```python
from build123d import *

# Parameters (mm, degrees)
REVOLUCI_N1_ANGLE       = 180
CROQUIS2_R              = 19
CORTAR_EXTRUIR1_DEPTH   = 29
SALIENTE_EXTRUIR1_DEPTH = 15
CROQUIS4_W              = 7
CROQUIS4_H              = 28
SALIENTE_EXTRUIR2_DEPTH = 10
CHAFL_N1_SIZE           = 5
REDONDEO1_R             = 10
CORTAR_EXTRUIR2_DEPTH   = 40


with BuildPart() as part:
    # Croquis1 → Revolución1 (revolve)
    with BuildSketch(Plane.XY):
        Polygon((0, 0), (0, 28), (25, 28), (25, 23), (22, 23), (22, 18), (25, 18), (25, 10), (22, 10), (22, 5), (25, 5), (25, 0), align=None)
    revolve(axis=Axis((0, 0, 0), (0, 1, 0)), revolution_arc=REVOLUCI_N1_ANGLE)

    # Croquis2 → Cortar-Extruir1 (cut)
    with BuildSketch(Plane(origin=(0, 28, 0), x_dir=(1, 0, 0), z_dir=(0, 1, 0))):
        Circle(CROQUIS2_R)
    extrude(amount=-CORTAR_EXTRUIR1_DEPTH, mode=Mode.SUBTRACT)

    # Croquis3 → Saliente-Extruir1 (add)
    with BuildSketch(Plane.XY):
        Polygon((25, 28), (24, 28), (24, 0), (31, 0), (31, 28), align=None)
    extrude(amount=-SALIENTE_EXTRUIR1_DEPTH)

    # Croquis4 → Saliente-Extruir2 (add)
    with BuildSketch(Plane.XY):
        with Locations((27.5, 14)):
            Rectangle(CROQUIS4_W, CROQUIS4_H)
    extrude(amount=SALIENTE_EXTRUIR2_DEPTH)

    # Chaflán1
    # the kernel refuses this chamfer: 5 mm, written as the material it adds along each edge
    with BuildSketch(Plane(origin=(24, 10.14158506, 0), x_dir=(0.027495876610586317, 0, 0.9996219169112968), z_dir=(0, 1, 0))) as chafl_n1_piece_1_section:
        Polygon((CHAFL_N1_SIZE * 0.999621916911, -CHAFL_N1_SIZE * 0.0274958766106), (-CHAFL_N1_SIZE * 0.0274958766106, -CHAFL_N1_SIZE * 0.999621916911), (0, 0), align=None)
    chafl_n1_piece_1 = extrude(amount=30.71682988, mode=Mode.PRIVATE)
    chafl_n1_piece_1 = split(chafl_n1_piece_1, bisect_by=Plane(origin=(23.057401275, 18, 2.044863286), z_dir=(0, -1, 0)), keep=Keep.TOP, mode=Mode.PRIVATE)
    add(chafl_n1_piece_1)
    with BuildSketch(Plane(origin=(24, 10.14158506, 0), x_dir=(0.027495876610586317, 0, 0.9996219169112968), z_dir=(0, 1, 0))) as chafl_n1_piece_2_section:
        Polygon((CHAFL_N1_SIZE * 0.999621916911, -CHAFL_N1_SIZE * 0.0274958766106), (-CHAFL_N1_SIZE * 0.0274958766106, -CHAFL_N1_SIZE * 0.999621916911), (0, 0), align=None)
    chafl_n1_piece_2 = extrude(amount=17.85841494, mode=Mode.PRIVATE)
    chafl_n1_piece_2 = chafl_n1_piece_2 & Plane(origin=(0, 20.5, 0), x_dir=(1, 0, 0), z_dir=(0, -1, 0)) * Cylinder(22, 56, mode=Mode.PRIVATE)
    add(chafl_n1_piece_2)
    with BuildSketch(Plane(origin=(24, 23, 0), x_dir=(0.027495876610586317, 0, 0.9996219169112968), z_dir=(0, 1, 0)), Plane(origin=(24, 0, 0), x_dir=(0.027495876610586317, 0, 0.9996219169112968), z_dir=(0, 1, 0))) as chafl_n1_piece_3:
        Polygon((CHAFL_N1_SIZE * 0.999621916911, -CHAFL_N1_SIZE * 0.0274958766106), (-CHAFL_N1_SIZE * 0.0274958766106, -CHAFL_N1_SIZE * 0.999621916911), (0, 0), align=None)
    extrude(amount=5)
    with BuildSketch(Plane(origin=(24, -2.85841494, 0), x_dir=(0.027495876610586317, 0, 0.9996219169112968), z_dir=(0, 1, 0))) as chafl_n1_piece_4_section:
        Polygon((CHAFL_N1_SIZE * 0.999621916911, -CHAFL_N1_SIZE * 0.0274958766106), (-CHAFL_N1_SIZE * 0.0274958766106, -CHAFL_N1_SIZE * 0.999621916911), (0, 0), align=None)
    chafl_n1_piece_4 = extrude(amount=33.71682988, mode=Mode.PRIVATE)
    chafl_n1_piece_4 = split(chafl_n1_piece_4, bisect_by=Plane(origin=(23.057401275, 0, 2.044863286), z_dir=(0, 1, 0)), keep=Keep.TOP, mode=Mode.PRIVATE)
    chafl_n1_piece_4 = split(chafl_n1_piece_4, bisect_by=Plane(origin=(23.057401275, 5, 2.044863286), z_dir=(0, -1, 0)), keep=Keep.TOP, mode=Mode.PRIVATE)
    add(chafl_n1_piece_4)
    with BuildSketch(Plane(origin=(24, -2.85841494, 0), x_dir=(0.027495876610586317, 0, 0.9996219169112968), z_dir=(0, 1, 0))) as chafl_n1_piece_5_section:
        Polygon((CHAFL_N1_SIZE * 0.999621916911, -CHAFL_N1_SIZE * 0.0274958766106), (-CHAFL_N1_SIZE * 0.0274958766106, -CHAFL_N1_SIZE * 0.999621916911), (0, 0), align=None)
    chafl_n1_piece_5 = extrude(amount=33.71682988, mode=Mode.PRIVATE)
    chafl_n1_piece_5 = split(chafl_n1_piece_5, bisect_by=Plane(origin=(20.959134142, 28, 0.94889219), z_dir=(0, -1, 0)), keep=Keep.TOP, mode=Mode.PRIVATE)
    chafl_n1_piece_5 = split(chafl_n1_piece_5, bisect_by=Plane(origin=(20.959134142, 5, 0.94889219), z_dir=(0, 1, 0)), keep=Keep.TOP, mode=Mode.PRIVATE)
    chafl_n1_piece_5 = chafl_n1_piece_5 & Plane(origin=(0, 7.5, 0), x_dir=(1, 0, 0), z_dir=(0, -1, 0)) * Cylinder(22, 88, mode=Mode.PRIVATE)
    add(chafl_n1_piece_5)
    with BuildSketch(Plane(origin=(24, 10, 0), x_dir=(0.027495876610586317, 0, 0.9996219169112968), z_dir=(0, 1, 0))) as chafl_n1_piece_6:
        Polygon((CHAFL_N1_SIZE * 0.999621916911, -CHAFL_N1_SIZE * 0.0274958766106), (-CHAFL_N1_SIZE * 0.0274958766106, -CHAFL_N1_SIZE * 0.999621916911), (0, 0), align=None)
    extrude(amount=8)
    with BuildSketch(Plane(origin=(24, -2.85841494, 0), x_dir=(0.027495876610586317, 0, 0.9996219169112968), z_dir=(0, 1, 0))) as chafl_n1_piece_7_section:
        Polygon((CHAFL_N1_SIZE * 0.999621916911, -CHAFL_N1_SIZE * 0.0274958766106), (-CHAFL_N1_SIZE * 0.0274958766106, -CHAFL_N1_SIZE * 0.999621916911), (0, 0), align=None)
    chafl_n1_piece_7 = extrude(amount=33.71682988, mode=Mode.PRIVATE)
    chafl_n1_piece_7 = split(chafl_n1_piece_7, bisect_by=Plane(origin=(23.057401275, 28, 2.044863286), z_dir=(0, -1, 0)), keep=Keep.TOP, mode=Mode.PRIVATE)
    chafl_n1_piece_7 = split(chafl_n1_piece_7, bisect_by=Plane(origin=(23.057401275, 23, 2.044863286), z_dir=(0, 1, 0)), keep=Keep.TOP, mode=Mode.PRIVATE)
    add(chafl_n1_piece_7)
    with BuildSketch(Plane(origin=(24, -12.85841494, 0), x_dir=(0.027495876610586317, 0, 0.9996219169112968), z_dir=(0, 1, 0))) as chafl_n1_piece_8_section:
        Polygon((CHAFL_N1_SIZE * 0.999621916911, -CHAFL_N1_SIZE * 0.0274958766106), (-CHAFL_N1_SIZE * 0.0274958766106, -CHAFL_N1_SIZE * 0.999621916911), (0, 0), align=None)
    chafl_n1_piece_8 = extrude(amount=30.71682988, mode=Mode.PRIVATE)
    chafl_n1_piece_8 = split(chafl_n1_piece_8, bisect_by=Plane(origin=(20.959134142, 5, 0.94889219), z_dir=(0, 1, 0)), keep=Keep.TOP, mode=Mode.PRIVATE)
    chafl_n1_piece_8 = chafl_n1_piece_8 & Plane(origin=(0, 7.5, 0), x_dir=(1, 0, 0), z_dir=(0, -1, 0)) * Cylinder(22, 82, mode=Mode.PRIVATE)
    add(chafl_n1_piece_8)
    with BuildSketch(Plane(origin=(24, -12.85841494, 0), x_dir=(0.027495876610586317, 0, 0.9996219169112968), z_dir=(0, 1, 0))) as chafl_n1_piece_9_section:
        Polygon((CHAFL_N1_SIZE * 0.999621916911, -CHAFL_N1_SIZE * 0.0274958766106), (-CHAFL_N1_SIZE * 0.0274958766106, -CHAFL_N1_SIZE * 0.999621916911), (0, 0), align=None)
    chafl_n1_piece_9 = extrude(amount=30.71682988, mode=Mode.PRIVATE)
    chafl_n1_piece_9 = split(chafl_n1_piece_9, bisect_by=Plane(origin=(23.057401275, 10, 2.044863286), z_dir=(0, 1, 0)), keep=Keep.TOP, mode=Mode.PRIVATE)
    add(chafl_n1_piece_9)

    # Redondeo1
    # the kernel refuses this fillet: 10 mm, written as the material it adds along each edge
    with BuildSketch(Plane(origin=(24, 28, -7), x_dir=(-0.5136512800645924, 0, -0.8579990457384005), z_dir=(0, -1, 0)), Plane(origin=(24, 5, -7), x_dir=(-0.5136512800645924, 0, -0.8579990457384005), z_dir=(0, -1, 0))) as redondeo1_piece_1:
        with BuildLine():
            CenterArc((15.171929763, 9.675014423), REDONDEO1_R, 213.819639199, 41.5332183)
            Line((6.863992366, 4.109210241), (0, 0))
            ThreePointArc((0, 0), (6.321637401, 0.812463942), (12.643274803, 0))
        make_face()
    extrude(amount=5)
    with BuildSketch(Plane(origin=(24, 59.608187007, -7), x_dir=(-0.5136512800645924, 0, -0.8579990457384005), z_dir=(0, -1, 0))) as redondeo1_piece_2_section:
        with BuildLine():
            CenterArc((15.171929763, 9.675014423), REDONDEO1_R, 213.819639199, 41.5332183)
            Line((6.863992366, 4.109210241), (0, 0))
            ThreePointArc((0, 0), (6.321637401, 0.812463942), (12.643274803, 0))
        make_face()
    redondeo1_piece_2 = extrude(amount=68.216374014, mode=Mode.PRIVATE)
    redondeo1_piece_2 = split(redondeo1_piece_2, bisect_by=Plane(origin=(20.483934171, 18, -15.810663128), z_dir=(0, -1, 0)), keep=Keep.TOP, mode=Mode.PRIVATE)
    redondeo1_piece_2 = split(redondeo1_piece_2, bisect_by=Plane(origin=(20.483934171, 10, -15.810663128), z_dir=(0, 1, 0)), keep=Keep.TOP, mode=Mode.PRIVATE)
    add(redondeo1_piece_2)
    with BuildSketch(Plane(origin=(24, 59.608187007, -7), x_dir=(-0.5136512800645924, 0, -0.8579990457384005), z_dir=(0, -1, 0))) as redondeo1_piece_3_section:
        with BuildLine():
            CenterArc((15.171929763, 9.675014423), REDONDEO1_R, 213.819639199, 41.5332183)
            Line((6.863992366, 4.109210241), (0, 0))
            ThreePointArc((0, 0), (6.321637401, 0.812463942), (12.643274803, 0))
        make_face()
    redondeo1_piece_3 = extrude(amount=68.216374014, mode=Mode.PRIVATE)
    redondeo1_piece_3 = split(redondeo1_piece_3, bisect_by=Plane(origin=(20.483934171, 5, -15.810663128), z_dir=(0, -1, 0)), keep=Keep.TOP, mode=Mode.PRIVATE)
    redondeo1_piece_3 = split(redondeo1_piece_3, bisect_by=Plane(origin=(20.483934171, 0, -15.810663128), z_dir=(0, 1, 0)), keep=Keep.TOP, mode=Mode.PRIVATE)
    add(redondeo1_piece_3)
    with BuildSketch(Plane(origin=(24, 49.608187007, -7), x_dir=(-0.5136512800645924, 0, -0.8579990457384005), z_dir=(0, -1, 0))) as redondeo1_piece_4_section:
        with BuildLine():
            CenterArc((15.171929763, 9.675014423), REDONDEO1_R, 213.819639199, 41.5332183)
            Line((6.863992366, 4.109210241), (0, 0))
            ThreePointArc((0, 0), (6.321637401, 0.812463942), (12.643274803, 0))
        make_face()
    redondeo1_piece_4 = extrude(amount=71.216374014, mode=Mode.PRIVATE)
    redondeo1_piece_4 = split(redondeo1_piece_4, bisect_by=Plane(origin=(20.483934171, 28, -15.810663128), z_dir=(0, -1, 0)), keep=Keep.TOP, mode=Mode.PRIVATE)
    redondeo1_piece_4 = split(redondeo1_piece_4, bisect_by=Plane(origin=(20.483934171, 23, -15.810663128), z_dir=(0, 1, 0)), keep=Keep.TOP, mode=Mode.PRIVATE)
    add(redondeo1_piece_4)
    with BuildSketch(Plane(origin=(24, 18, -7), x_dir=(-0.5136512800645924, 0, -0.8579990457384005), z_dir=(0, -1, 0))) as redondeo1_piece_5:
        with BuildLine():
            CenterArc((15.171929763, 9.675014423), REDONDEO1_R, 213.819639199, 41.5332183)
            Line((6.863992366, 4.109210241), (0, 0))
            ThreePointArc((0, 0), (6.321637401, 0.812463942), (12.643274803, 0))
        make_face()
    extrude(amount=8)
    with BuildSketch(Plane(origin=(24, 49.608187007, -7), x_dir=(-0.5136512800645924, 0, -0.8579990457384005), z_dir=(0, -1, 0))) as redondeo1_piece_6_section:
        with BuildLine():
            CenterArc((15.171929763, 9.675014423), REDONDEO1_R, 213.819639199, 41.5332183)
            Line((6.863992366, 4.109210241), (0, 0))
            ThreePointArc((0, 0), (6.321637401, 0.812463942), (12.643274803, 0))
        make_face()
    redondeo1_piece_6 = extrude(amount=71.216374014, mode=Mode.PRIVATE)
    redondeo1_piece_6 = split(redondeo1_piece_6, bisect_by=Plane(origin=(20.483934171, 5, -15.810663128), z_dir=(0, -1, 0)), keep=Keep.TOP, mode=Mode.PRIVATE)
    redondeo1_piece_6 = split(redondeo1_piece_6, bisect_by=Plane(origin=(20.483934171, 0, -15.810663128), z_dir=(0, 1, 0)), keep=Keep.TOP, mode=Mode.PRIVATE)
    add(redondeo1_piece_6)
    with BuildSketch(Plane(origin=(24, 36.608187007, -7), x_dir=(-0.5136512800645924, 0, -0.8579990457384005), z_dir=(0, -1, 0))) as redondeo1_piece_7_section:
        with BuildLine():
            CenterArc((15.171929763, 9.675014423), REDONDEO1_R, 213.819639199, 41.5332183)
            Line((6.863992366, 4.109210241), (0, 0))
            ThreePointArc((0, 0), (6.321637401, 0.812463942), (12.643274803, 0))
        make_face()
    redondeo1_piece_7 = extrude(amount=68.216374014, mode=Mode.PRIVATE)
    redondeo1_piece_7 = split(redondeo1_piece_7, bisect_by=Plane(origin=(20.483934171, 28, -15.810663128), z_dir=(0, -1, 0)), keep=Keep.TOP, mode=Mode.PRIVATE)
    redondeo1_piece_7 = split(redondeo1_piece_7, bisect_by=Plane(origin=(20.483934171, 23, -15.810663128), z_dir=(0, 1, 0)), keep=Keep.TOP, mode=Mode.PRIVATE)
    add(redondeo1_piece_7)
    with BuildSketch(Plane(origin=(24, 36.608187007, -7), x_dir=(-0.5136512800645924, 0, -0.8579990457384005), z_dir=(0, -1, 0))) as redondeo1_piece_8_section:
        with BuildLine():
            CenterArc((15.171929763, 9.675014423), REDONDEO1_R, 213.819639199, 41.5332183)
            Line((6.863992366, 4.109210241), (0, 0))
            ThreePointArc((0, 0), (6.321637401, 0.812463942), (12.643274803, 0))
        make_face()
    redondeo1_piece_8 = extrude(amount=68.216374014, mode=Mode.PRIVATE)
    redondeo1_piece_8 = split(redondeo1_piece_8, bisect_by=Plane(origin=(20.483934171, 18, -15.810663128), z_dir=(0, -1, 0)), keep=Keep.TOP, mode=Mode.PRIVATE)
    redondeo1_piece_8 = split(redondeo1_piece_8, bisect_by=Plane(origin=(20.483934171, 10, -15.810663128), z_dir=(0, 1, 0)), keep=Keep.TOP, mode=Mode.PRIVATE)
    add(redondeo1_piece_8)

    # Croquis5 → Cortar-Extruir2 (cut)
    with BuildSketch(Plane(origin=(0, 0, -15), x_dir=(-1, 0, 0), z_dir=(0, 0, -1))):
        Polygon((-31, 14), (-31, 11), (-28, 11), (-28, 17), (-31, 17), align=None)
    extrude(amount=-CORTAR_EXTRUIR2_DEPTH, mode=Mode.SUBTRACT)


solid = part.part
```
Part model, mm, in its own coordinate system. A direction names the side the tool comes from. Round coordinates to 2 decimals unless told otherwise and drop trailing zeros. Write each loop counter-clockwise with the first axis right and the second up, starting at its lowest first coordinate (ties: lowest second). Pieces come first, ordered by that corner, then holes. Notation, with made-up numbers: M 3,55.5 L 44,55.5 A28 cw 44,91.5 Z; hole C -37,-39 d5. An arc over 180 degrees is marked long. Answer as CSV lines item,"result". Start each with the question number.
1) Mould opens along Y. For faces 5 (the face through (29, 17, -3)), 6 (the face through (13.2, 0, -14.1)), 7 (the face through (-9.299, 13.944, -23.206)), 8 (the face through (14.2, 28, -13.2)) say: +Y half, -Y half, draft (parallel to the pull), parting line (faces both ways), or undercut.
2) Band-saw the part on C-C (x = 0). List the corners of the cut face in (y, z).
3) Which spindle directions (+Z, -Z, +X, -X, +Y, -Y) get a long thin tool onto all of the face, cutting with end or side? Do faces 1 (the face through (-9.299, 25.465, -23.206)), 2 (the face through (3, 5, -22)), 3 (the face through (24, 14, 6)), 4 (the face through (30, 11, -3)). Say none if no direction does.
4) Band-saw the part on B-B (y = 7). List the corners of the cut face in (x, z).
5) Band-saw the part on A-A (z = -1). List the corners of the cut face in (x, y).
6) Band-saw the part on D-D (z = -16). List the corners of the cut face in (x, y), then the cut area to 3 significant figures.
7) Drop flat-ended pins along their axis: pin 1 (12 mm diameter, centred on x = 0, y = 23.5, fed in from +Z); pin 2 (4 mm diameter, centred on y = 10.5, z = -6.5, fed in from -X); pin 3 (2 mm diameter, centred on x = 27, y = 19.5, fed in from -Z). Give the stop position or say it passes through.
8) Drill centre lines: L1, parallel to Y at x = 6.5, z = -23; L2, parallel to X at y = 7, z = -0.5; L3, parallel to X at y = 8, z = -13. Where is each one in solid material? Low to high.
Worked out:
1,face 5,"undercut"
1,face 6,"-Y half"
1,face 7,"draft"
1,face 8,"+Y half"
2,outline,"M 0,-25 L 5,-25 L 5,-22 L 10,-22 L 10,-25 L 18,-25 L 18,-22 L 23,-22 L 23,-25 L 28,-25 L 28,-19 L 0,-19 Z"
3,face 1,"-Z, +Y, -Y"
3,face 2,"-Z"
3,face 3,"+Z"
3,face 4,"+Z, -Z, +X"
4,outline,"M -22,0 A22 ccw long 21.82,2.82 L 19,0 A19 cw -19,0 Z; M 24,-15 L 31,-15 L 31,10 L 24,10 Z"
5,outline,"M -24.98,0 L -18.97,0 L -18.97,28 L -24.98,28 L -24.98,23 L -21.98,23 L -21.98,18 L -24.98,18 L -24.98,10 L -21.98,10 L -21.98,5 L -24.98,5 Z; M 18.97,0 L 31,0 L 31,11 L 28,11 L 28,17 L 31,17 L 31,28 L 18.97,28 Z; hole M 21.98,5 L 24,5 L 24,10 L 21.98,10 Z; hole M 21.98,18 L 24,18 L 24,23 L 21.98,23 Z"
6,outline,"M -19.21,0 L -10.25,0 L -10.25,28 L -19.21,28 L -19.21,23 L -15.1,23 L -15.1,18 L -19.21,18 L -19.21,10 L -15.1,10 L -15.1,5 L -19.21,5 Z; M 10.25,0 L 20.12,0 L 20.12,5 L 15.1,5 L 15.1,10 L 20.12,10 L 20.12,18 L 15.1,18 L 15.1,23 L 20.12,23 L 20.12,28 L 10.25,28 Z"
6,area,"436 mm²"
7,pin 1,"z = -18.03"
7,pin 2,"x = -24.59"
7,pin 3,"z = -15"
8,L1,"0 to 5, 10 to 18, 23 to 28"
8,L2,"-21.99 to -18.99, 18.99 to 21.99, 24 to 31"
8,L3,"-17.75 to -13.86, 13.86 to 17.75, 24 to 31"
